For this review, take the finished solid that the model builds, in its own axes (mm). Round coordinates to 2 decimals unless told otherwise and drop trailing zeros. Write each loop counter-clockwise with the first axis right and the second up, starting at its lowest first coordinate (ties: lowest second). Pieces come first, ordered by that corner, then holes. Notation, with made-up numbers: (22.25, 82.25) -> (31.25, 82.25) arc R28 ccw to (31.25, 121.25) -> close; hole circle Ø10 at (89.5, 89.5). An arc over 180 degrees is marked (long way). Answer in a Markdown table with one row per item.
from build123d import *

# Parameters (mm, degrees)
SKETCH1_R               = 38.1
SKETCH1_R_2             = 31.75
BOSS_EXTRUDE1_DEPTH     = 25.4
CUT_EXTRUDE1_START      = -10
SKETCH2_R               = 2
CUT_EXTRUDE1_DEPTH      = 99.9
CIRPATTERN1_START       = 31.686945161
CIRPATTERN1_OUTLINE_R   = 2
CIRPATTERN1_DEPTH       = 6.413054905
CIRPATTERN1_START_2     = -38.100000066
CIRPATTERN1_2_OUTLINE_R = 2
CIRPATTERN1_2_DEPTH     = 76.200000132


# Read off the part's stored shape, not the designer's step: CirPattern1
with BuildPart() as part:
    # Sketch1 → Boss-Extrude1 (new body)
    with BuildSketch(Plane(origin=(0, 0, 0), x_dir=(1, 0, 0), z_dir=(0, 1, 0))):
        with Locations(Location((0, 0, 0), (0, 0, 270))):
            Circle(SKETCH1_R)
        with Locations(Location((0, 0, 0), (0, 0, 270))):
            Circle(SKETCH1_R_2, mode=Mode.SUBTRACT)
    extrude(amount=BOSS_EXTRUDE1_DEPTH)

    # Sketch2 → Cut-Extrude1 (cut)
    with BuildSketch(Plane.ZY.offset(38.1).offset(CUT_EXTRUDE1_START)):
        with Locations(Location((0, 15.24, 0), (0, 0, 180))):
            Circle(SKETCH2_R)
    extrude(amount=CUT_EXTRUDE1_DEPTH, mode=Mode.SUBTRACT)

    # CirPattern1 outline → CirPattern1 (cut)
    with BuildSketch(Plane.YZ.offset(CIRPATTERN1_START)):
        with Locations((15.24, 0)):
            Circle(CIRPATTERN1_OUTLINE_R)
    extrude(amount=CIRPATTERN1_DEPTH, mode=Mode.SUBTRACT)

    # CirPattern1 2 outline → CirPattern1 2 (cut)
    with BuildSketch(Plane.XY.offset(CIRPATTERN1_START_2)):
        with Locations((0, 15.24)):
            Circle(CIRPATTERN1_2_OUTLINE_R)
    extrude(amount=CIRPATTERN1_2_DEPTH, mode=Mode.SUBTRACT)


solid = part.part
1) Clearance check with flat-ended pins moving along their axes: pin 1 Ø4 at (y, z) = (6.5, -6) entering from +X; pin 2 Ø3 at (x, z) = (-22.5, 23.5) entering from -Y; pin 3 Ø8 at (x, y) = (11, 8) entering from +Z; pin 4 Ø5 at (y, z) = (22.5, 21) entering from +X. State where each tip first meets the part, or that it passes through.
Solved:
| item | result |
|---|---|
| pin 1 | x = 37.89 |
| pin 2 | y = 0 |
| pin 3 | z = 37.45 |
| pin 4 | x = 33.31 |
2) Consider section C-C on x = 19.5. State the section outline as (y, z) points, then the cut area to 3 significant figures.
Solved:
| item | result |
|---|---|
| outline | (0, -32.73) -> (25.4, -32.73) -> (25.4, -25.06) -> (0, -25.06) -> close; (0, 25.06) -> (25.4, 25.06) -> (25.4, 32.73) -> (0, 32.73) -> close |
| area | 390 mm² |
3) Consider section B-B on z = 13. State the section outline as (x, y) points, then the cut area to 3 significant figures.
Solved:
| item | result |
|---|---|
| outline | (-35.81, 0) -> (-28.97, 0) -> (-28.97, 25.4) -> (-35.81, 25.4) -> close; (28.97, 0) -> (35.81, 0) -> (35.81, 25.4) -> (28.97, 25.4) -> close |
| area | 348 mm² |
4) Mouldability with a two-part tool opening along Y and no side actions: class faces 1 (the flat face through (31, 0, -9)), 2 (the cylindrical face through (-0.26, 17.223, -34.938)), 3 (the flat face through (31, 25.4, -9)) as pulls with the +Y half, pulls with the -Y half, needs draft (parallel to the pull), parting line crosses it, or undercut.
Solved:
| item | result |
|---|---|
| face 1 | pulls with the -Y half |
| face 2 | undercut |
| face 3 | pulls with the +Y half |
5) Consider section A-A on x = 0. State the section outline as (y, z) points.
Solved:
| item | result |
|---|---|
| outline | (0, -38.1) -> (13.24, -38.1) -> (13.24, -31.75) -> (0, -31.75) -> close; (0, 31.75) -> (13.24, 31.75) -> (13.24, 38.1) -> (0, 38.1) -> close; (17.24, -38.1) -> (25.4, -38.1) -> (25.4, -31.75) -> (17.24, -31.75) -> close; (17.24, 31.75) -> (25.4, 31.75) -> (25.4, 38.1) -> (17.24, 38.1) -> close |
6) For line 1 (Y direction, x = 34, z = 0); line 2 (Z direction, x = -1.5, y = 13.5); line 3 (Z direction, x = -27.5, y = 19), list the stretches that pass through material, from the lowest coordinate up. Write a range as [from, to].
Solved:
| item | result |
|---|---|
| line 1 | [0, 13.24], [17.24, 25.4] |
| line 2 | [-38.07, -31.71], [31.71, 38.07] |
| line 3 | [-26.37, -15.87], [15.87, 26.37] |
7) Consider section D-D on y = 15.24. State the section outline as (x, z) points.
Solved:
| item | result |
|---|---|
| outline | (-38.05, -2) arc R38.1 ccw to (-2, -38.05) -> (-2, -31.69) arc R31.75 cw to (-31.69, -2) -> close; (-38.05, 2) -> (-31.69, 2) arc R31.75 cw to (-2, 31.69) -> (-2, 38.05) arc R38.1 ccw to start; (2, -38.05) arc R38.1 ccw to (38.05, -2) -> (31.69, -2) arc R31.75 cw to (2, -31.69) -> close; (2, 31.69) arc R31.75 cw to (31.69, 2) -> (38.05, 2) arc R38.1 ccw to (2, 38.05) -> close |
